Model file for the job. Use its own axes, mm. A direction names the side the tool comes from. Coordinates: 2 decimals unless noted, no trailing zeros. Write each loop counter-clockwise with the first axis right and the second up, starting at its lowest first coordinate (ties: lowest second). Pieces come first, ordered by that corner, then holes. Notation, with made-up numbers: (71.5, -2) - (111.5, -2) arc R26 cw to (111.5, 23) - close; hole circle Ø4 at (60, 46). An arc over 180 degrees is marked (long way). Put each result on its own line as item: value. Start each with the question number.
1. Drop flat-ended pins along their axis: P1, Ø8, axis at x = 15.5, y = -8, coming from the +Z side; P2, Ø2, axis at x = 6, y = -18.5, coming from the -Z side; P3, Ø5, axis at y = -14, z = -10.5, coming from the +X side. Give the stop position or say it passes through.
2. Pull direction X, two halves, no side cores. Call faces 5 (the face through (22, -25, -11)), 6 (the face through (23.522, -45, -12)), 7 (the face through (14, -32, -5.6)): released by +X, released by -X, zero draft, split by the parting line, or undercut.
3. Which spindle directions (+Z, -Z, +X, -X, +Y, -Y) get a long thin tool onto all of the face, cutting with end or side? Do faces 1 (the face through (13, -12, -19.6)), 2 (the face through (21.522, -12, -12)), 3 (the face through (7.522, -32, -12)), 4 (the face through (5.522, -12, -12)). Say none if no direction does.
4. Saw through at C-C, the plane x = 10. Write the cut outline in (y, z).
5. Saw through at A-A, the plane z = -8. Write the cut outline in (x, y).
6. Saw through at D-D, the plane y = -12.5. Write the cut outline in (x, z).
7. Drill centre lines: L1, parallel to Z at x = 15.25, y = -44; L2, parallel to X at y = -48, z = -10.75; L3, parallel to X at y = -20.5, z = -11.5. Where is each one in solid material? Low to high. Write a range as from..to.
8. Saw through at B-B, the plane y = -24. Write the cut outline in (x, z), plus the area to 3 significant figures.
```python
from build123d import *

# Parameters (mm, degrees)
F0_W     = 16
F0_H     = 16
F1_DEPTH = 25
F2_W     = 12
F2_H     = 12
F3_DEPTH = 25
F4_W     = 20
F4_H     = 20
F5_DEPTH = 40
F6_R     = 5
F7_DEPTH = 2
F8_W     = 12
F8_H     = 12
F9_DEPTH = 40


with BuildPart() as f1:
    # F0 (on Front) → F1 (new body)
    with BuildSketch(Plane.XZ):
        with Locations((13.521624, -11.600108)):
            Rectangle(F0_W, F0_H)
    extrude(amount=F1_DEPTH)

    # F2 (on face) → F3 (cut)
    with BuildSketch(Plane(origin=(0, 0, 0), x_dir=(-1, 0, 0), z_dir=(0, 1, 0))):
        with Locations((-13.521624, -11.600108)):
            Rectangle(F2_W, F2_H)
    extrude(amount=-F3_DEPTH, mode=Mode.SUBTRACT)

    # F4 (on face) → F5 (join)
    with BuildSketch(Plane.XZ.offset(25)):
        with Locations((13.521624, -11.600108)):
            Rectangle(F4_W, F4_H)
    extrude(amount=F5_DEPTH)

    # F6 (on face) → F7 (cut, through all)
    with BuildSketch(Plane.XY.offset(-3.600108)):
        with Locations((13.521624, -12.5)):
            Circle(F6_R)
    extrude(amount=-F7_DEPTH, mode=Mode.SUBTRACT)

    # F8 (on face) → F9 (cut, through all)
    with BuildSketch(Plane(origin=(0, -25, 0), x_dir=(-1, 0, 0), z_dir=(0, 1, 0))):
        with Locations((-13.521624, -11.600108)):
            Rectangle(F8_W, F8_H)
    extrude(amount=-F9_DEPTH, mode=Mode.SUBTRACT)


solid = f1.part
```
Final values:
1. P1: stops at z = -3.6
1. P2: stops at z = -19.6
1. P3: stops at x = 21.52
2. face 5: zero draft
2. face 6: released by +X
2. face 7: undercut
3. face 1: -Z, +X, -X, +Y
3. face 2: +Z, -Z, +X, +Y
3. face 3: +Y, -Y
3. face 4: +Z, -Z, -X, +Y
4. outline: (-65, -21.6) - (-25, -21.6) - (-25, -19.6) - (0, -19.6) - (0, -17.6) - (-65, -17.6) - close; (-65, -5.6) - (-16.05, -5.6) - (-16.05, -3.6) - (-25, -3.6) - (-25, -1.6) - (-65, -1.6) - close; (-8.95, -5.6) - (0, -5.6) - (0, -3.6) - (-8.95, -3.6) - close
5. outline: (3.52, -65) - (7.52, -65) - (7.52, 0) - (5.52, 0) - (5.52, -25) - (3.52, -25) - close; (19.52, -65) - (23.52, -65) - (23.52, -25) - (21.52, -25) - (21.52, 0) - (19.52, 0) - close
6. outline: (5.52, -19.6) - (21.52, -19.6) - (21.52, -3.6) - (18.52, -3.6) - (18.52, -5.6) - (19.52, -5.6) - (19.52, -17.6) - (7.52, -17.6) - (7.52, -5.6) - (8.52, -5.6) - (8.52, -3.6) - (5.52, -3.6) - close
7. L1: z = -21.6..-17.6, -5.6..-1.6
7. L2: x = 3.52..7.52, 19.52..23.52
7. L3: x = 5.52..7.52, 19.52..21.52
8. outline: (5.52, -19.6) - (21.52, -19.6) - (21.52, -3.6) - (5.52, -3.6) - close; hole (7.52, -17.6) - (19.52, -17.6) - (19.52, -5.6) - (7.52, -5.6) - close
8. area: 112 mm²
